For this review, use the dimensioned drawing (mm, ordinates from the lowest corner) and the shaded views. Round coordinates to 2 decimals unless told otherwise and drop trailing zeros. Write each loop counter-clockwise with the first axis right and the second up, starting at its lowest first coordinate (ties: lowest second). Pieces come first, ordered by that corner, then holes. Notation, with made-up numbers: (28, -9.75) - (80, -9.75) arc R26 cw to (80, 6.25) - close; hole circle Ø7 at (57, 27). An arc over 180 degrees is marked (long way). Return JSON: item names as keys, results as strings.
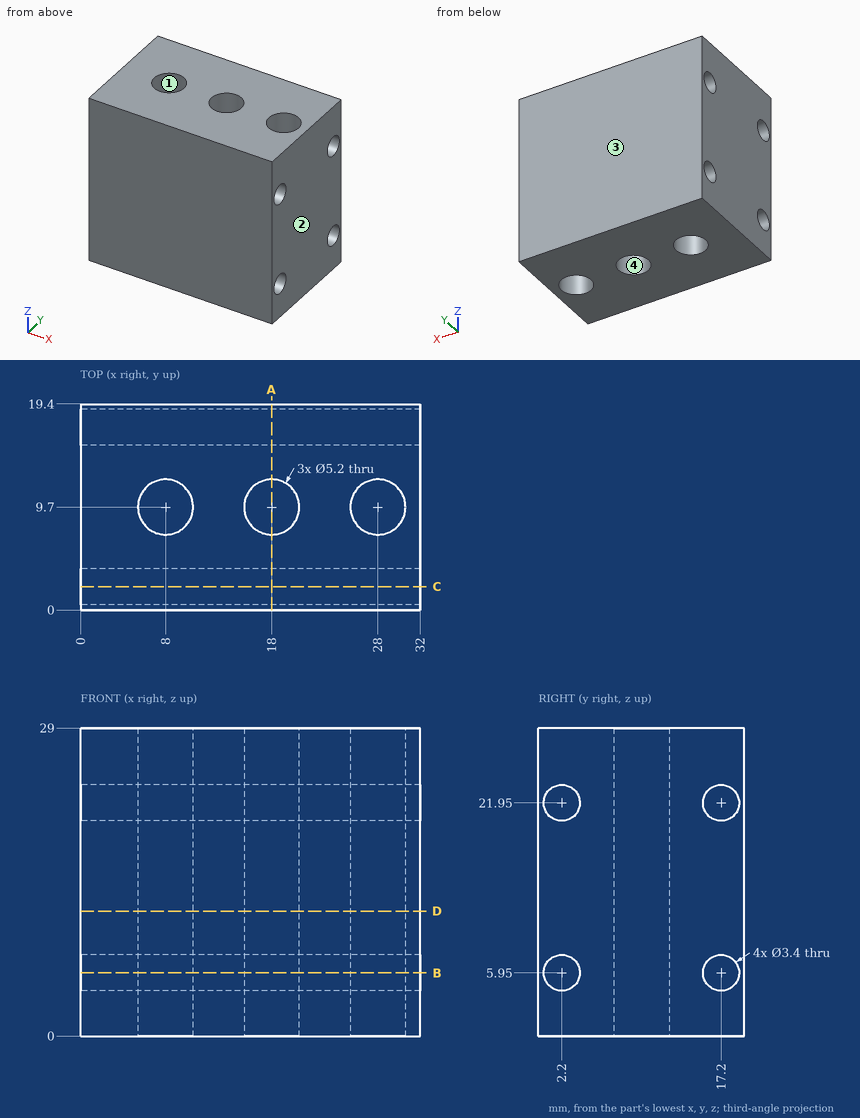
(1) Add section A-A (x = 18). Write out the cut boundary in (y, z), plus the area to 3 significant figures.
Filled in:
{"outline": "(0, 0) - (7.1, 0) - (7.1, 29) - (0, 29) - close; (12.3, 0) - (19.4, 0) - (19.4, 29) - (12.3, 29) - close; hole circle Ø3.4 at (2.2, 5.95); hole circle Ø3.4 at (2.2, 21.95); hole circle Ø3.4 at (17.2, 5.95); hole circle Ø3.4 at (17.2, 21.95)", "area": "375 mm2"}
(2) Add section D-D (z = 11.75). Write out the cut boundary in (x, y), plus the area to 3 significant figures.
Filled in:
{"outline": "(0, 0) - (32, 0) - (32, 19.4) - (0, 19.4) - close; hole circle Ø5.2 at (8, 9.7); hole circle Ø5.2 at (18, 9.7); hole circle Ø5.2 at (28, 9.7)", "area": "557 mm2"}
(3) Add section B-B (z = 5.95). Write out the cut boundary in (x, y), plus the area to 3 significant figures.
Filled in:
{"outline": "(0, 0) - (32, 0) - (32, 0.5) - (0, 0.5) - close; (0, 3.9) - (32, 3.9) - (32, 15.5) - (0, 15.5) - close; (0, 18.9) - (32, 18.9) - (32, 19.4) - (0, 19.4) - close; hole circle Ø5.2 at (8, 9.7); hole circle Ø5.2 at (18, 9.7); hole circle Ø5.2 at (28, 9.7)", "area": "339 mm2"}
(4) Add section C-C (y = 2.2). Write out the cut boundary in (x, z), plus the area to 3 significant figures.
Filled in:
{"outline": "(0, 0) - (32, 0) - (32, 4.25) - (0, 4.25) - close; (0, 7.65) - (32, 7.65) - (32, 20.25) - (0, 20.25) - close; (0, 23.65) - (32, 23.65) - (32, 29) - (0, 29) - close", "area": "710 mm2"}
(5) Wall thickness on line 1 (Y direction, x = 11, z = 5.95); line 2 (Z direction, x = 20.5, y = 17.25); line 3 (X direction, y = 11, z = 16): over which ranges is each line inside the solid? List them lowest first.
Filled in:
{"line 1": "y = 0 to 0.5, 3.9 to 15.5, 18.9 to 19.4", "line 2": "z = 0 to 4.25, 7.65 to 20.25, 23.65 to 29", "line 3": "x = 0 to 5.75, 10.25 to 15.75, 20.25 to 25.75, 30.25 to 32"}
(6) Clearance check with flat-ended pins moving along their axes: pin 1 Ø4 at (x, y) = (18, 9.7) entering from +Z; pin 2 Ø4.5 at (y, z) = (17.2, 5.95) entering from +X. State where each tip first meets the part, or that it passes through.
Filled in:
{"pin 1": "passes through", "pin 2": "stops at x = 32"}
(7) Mouldability with a two-part tool opening along X and no side actions: class the marked faces 1, 2, 3 and 4 as released by +X, released by -X, zero draft, split by the parting line, or undercut.
Filled in:
{"face 1": "undercut", "face 2": "released by +X", "face 3": "zero draft", "face 4": "undercut"}
